```python
from build123d import *

# Parameters (mm, degrees)
SKETCH1_R           = 1.5
BOSS_EXTRUDE1_DEPTH = 2


with BuildPart() as part:
    # Sketch1 → Boss-Extrude1 (new body)
    with BuildSketch(Plane.XY.offset(-1267.107479839)):
        with BuildLine():
            Line((36.146099055, 1376.306398419), (13.765371143, 1267.870458722))
            ThreePointArc((13.765371143, 1267.870458722), (12.991950286, 1262.843357254), (12.733250996, 1257.763691551))
            Line((12.733250996, 1257.763691551), (12.733250996, 1126.263691551))
            ThreePointArc((12.733250996, 1126.263691551), (15.662183185, 1119.192623739), (22.733250996, 1116.263691551))
            Line((22.733250996, 1116.263691551), (27.733250996, 1116.263691551))
            Line((27.733250996, 1116.263691551), (27.733250996, 1030.263691551))
            Line((27.733250996, 1030.263691551), (22.733250996, 1030.263691551))
            ThreePointArc((22.733250996, 1030.263691551), (15.662183185, 1027.334759363), (12.733250996, 1020.263691551))
            Line((12.733250996, 1020.263691551), (12.733250996, 999.263691551))
            ThreePointArc((12.733250996, 999.263691551), (15.662183185, 992.192623739), (22.733250996, 989.263691551))
            Line((22.733250996, 989.263691551), (358.733250996, 989.263691551))
            ThreePointArc((358.733250996, 989.263691551), (365.804318808, 992.192623739), (368.733250996, 999.263691551))
            Line((368.733250996, 999.263691551), (368.733250996, 1257.766155457))
            ThreePointArc((368.733250996, 1257.766155457), (368.437249077, 1263.198703185), (367.552748004, 1268.566929131))
            Line((367.552748004, 1268.566929131), (343.655165727, 1376.584001021))
            ThreePointArc((343.655165727, 1376.584001021), (336.649224027, 1387.858661724), (324.127366924, 1392.263691551))
            Line((324.127366924, 1392.263691551), (55.733250996, 1392.263691551))
            ThreePointArc((55.733250996, 1392.263691551), (43.101033008, 1387.769402392), (36.146099055, 1376.306398419))
        make_face()
        with Locations((19.733250996, 1010.263691551)):
            Circle(SKETCH1_R, mode=Mode.SUBTRACT)
        with Locations((62.733250996, 995.263691551)):
            Circle(SKETCH1_R, mode=Mode.SUBTRACT)
        with Locations((147.733250996, 995.263691551)):
            Circle(SKETCH1_R, mode=Mode.SUBTRACT)
        with Locations((233.733250996, 995.263691551)):
            Circle(SKETCH1_R, mode=Mode.SUBTRACT)
        with Locations((318.733250996, 995.263691551)):
            Circle(SKETCH1_R, mode=Mode.SUBTRACT)
        with Locations((361.733250996, 1051.263691551)):
            Circle(SKETCH1_R, mode=Mode.SUBTRACT)
        with Locations((361.733250996, 1131.263691551)):
            Circle(SKETCH1_R, mode=Mode.SUBTRACT)
        with Locations((361.733250996, 1211.263691551)):
            Circle(SKETCH1_R, mode=Mode.SUBTRACT)
        with Locations((355.36207357, 1291.263691551)):
            Circle(SKETCH1_R, mode=Mode.SUBTRACT)
        with Locations((342.401145161, 1349.84708796)):
            Circle(SKETCH1_R, mode=Mode.SUBTRACT)
        with Locations((293.655165727, 1385.263691551)):
            Circle(SKETCH1_R, mode=Mode.SUBTRACT)
        with Locations((223.655165727, 1385.263691551)):
            Circle(SKETCH1_R, mode=Mode.SUBTRACT)
        with Locations((156.146099055, 1385.263691551)):
            Circle(SKETCH1_R, mode=Mode.SUBTRACT)
        with Locations((86.146099055, 1385.263691551)):
            Circle(SKETCH1_R, mode=Mode.SUBTRACT)
        with Locations((39.065356832, 1349.84708796)):
            Circle(SKETCH1_R, mode=Mode.SUBTRACT)
        with Locations((26.104428423, 1291.263691551)):
            Circle(SKETCH1_R, mode=Mode.SUBTRACT)
        with Locations((19.733250996, 1216.263691551)):
            Circle(SKETCH1_R, mode=Mode.SUBTRACT)
        with Locations((19.733250996, 1136.263691551)):
            Circle(SKETCH1_R, mode=Mode.SUBTRACT)
    extrude(amount=BOSS_EXTRUDE1_DEPTH)


solid = part.part
```
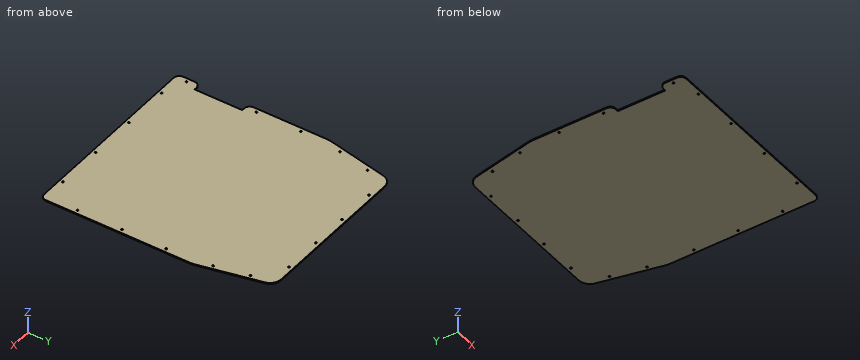
Geometry check sheet. Reference: the model listing, model coordinates, mm. Round coordinates to 2 decimals unless told otherwise and drop trailing zeros. Order: outer loops, then holes, each group sorted by start corner. A loop starts at its lowest first (then second) coordinate and runs counter-clockwise, first axis right, second up. Notation, with made-up numbers: M 0.5,5.5 L 6.5,5.5 A22 cw 6.5,16.5 Z; hole C -29,-4.5 d8. An arc over 180 degrees is marked long. Answer as CSV lines item,"result".
1) Thickness scan on probe 1 along X at (y, z) = (1292, -1265.9); probe 2 along Y at (x, z) = (293.5, -1266.95); probe 3 along Y at (x, z) = (224.5, -1266.3). Record the ranges inside material, lowest first. Write a range as [from, to].
Entries:
probe 1,"[18.75, 24.8], [27.41, 354.06], [356.67, 362.37]"
probe 2,"[989.26, 1383.77], [1386.76, 1392.26]"
probe 3,"[989.26, 1384.02], [1386.5, 1392.26]"
2) Sectioned sample at A-A on z = -1266.05. Give the number of separate pieces and of enclosed holes in the cut face, and give its area (3 significant figures).
Entries:
separate pieces,"1"
enclosed holes,"18"
area,"138,000 mm2"
3) Gauge pin test, flat end, axial feed: pin 1 Ø1 at (y, z) = (1080.5, -1266) entering from -X. Record the tip position at first contact, or that the pin passes through.
Entries:
pin 1,"x = 27.73"
4) Sectioned sample at C-C on y = 1098.5. Record the cut outline in (x, z).
Entries:
outline,"M 27.73,-1267.11 L 368.73,-1267.11 L 368.73,-1265.11 L 27.73,-1265.11 Z"
5) Sectioned sample at B-B on y = 1356. Record the cut outline in (x, z).
Entries:
outline,"M 31.95,-1267.11 L 348.21,-1267.11 L 348.21,-1265.11 L 31.95,-1265.11 Z"
